Source: CAD feature listing. Evaluate the final solid. Frame: model axes, mm. Face numbers are marked on the shaded views. A direction names the side the tool comes from. Coordinates: 2 decimals unless noted, no trailing zeros. Order: outer loops, then holes, each group sorted by start corner. A loop starts at its lowest first (then second) coordinate and runs counter-clockwise, first axis right, second up.
Item 1: Section B-B on y = 0. State how many separate pieces and enclosed holes the cut face has, then the cut area to 3 significant figures.
Item 2: Section A-A on z = 22. Return the cut outline in (x, y).
Item 3: Reachability of the marked faces 1, 2 and 3 from +Z, -Z, +X, -X, +Y, -Y: full face, straight path, thin tool, end or side. Return the list, or none.
Item 4: Ray query, line 1 (Z direction, x = 1.5, y = -0.75); line 2 (X direction, y = 0, z = 2.5); line 3 (Y direction, x = -1.5, z = 19.5). Return the intervals inside material, ascending.
Item 5: Contact query for flat-ended pins moving along their axis: P1, Ø4, axis at y = -1, z = 29, coming from the +X side; P2, Ø0.6, axis at y = 1.5, z = 40, coming from the -X side; P3, Ø2.5, axis at x = 0, y = 0, coming from the -Z side; P4, Ø0.6, axis at x = 1, y = -2, coming from the -Z side. Output: stop coordinate, or through.
from build123d import *

# Parameters (mm, degrees)
SKETCH_R        = 2.5
SKETCH_R_2      = 1.6
PAD_DEPTH       = 45
PAD001_DEPTH    = 1.5
PAD002_DEPTH    = 5
SKETCH003_W     = 2
SKETCH003_H     = 7
POCKET_DEPTH    = 7.001
SKETCH004_R     = 1.1
POCKET001_DEPTH = 7.001
SKETCH006_W     = 2.5
SKETCH006_H     = 6.5
POCKET002_DEPTH = 8.001
SKETCH005_W     = 2.5
SKETCH005_H     = 6
POCKET003_DEPTH = 8.001
POCKET004_DEPTH = 7.001


with BuildPart() as part:
    # Sketch → Pad (new body)
    with BuildSketch(Plane.XY):
        Circle(SKETCH_R)
        Circle(SKETCH_R_2, mode=Mode.SUBTRACT)
    extrude(amount=PAD_DEPTH)

    # Sketch001 (on Face3 of Pad) → Pad001 (join)
    with BuildSketch(Plane(origin=(0, 0, 7), x_dir=(1, 0, 0), z_dir=(0, 0, -1))):
        with BuildLine():
            Line((-2, 4), (2, 4))
            ThreePointArc((4, 2), (3.414214, 3.414214), (2, 4))
            Line((4, 2), (4, -2))
            ThreePointArc((2, -4), (3.414214, -3.414214), (4, -2))
            Line((2, -4), (-2, -4))
            ThreePointArc((-4, -2), (-3.414214, -3.414214), (-2, -4))
            Line((-4, -2), (-4, 2))
            ThreePointArc((-2, 4), (-3.414214, 3.414214), (-4, 2))
        make_face()
    extrude(amount=-PAD001_DEPTH)

    # Sketch002 (on Face16 of Pad001) → Pad002 (join)
    with BuildSketch(Plane.XY.offset(45)):
        with BuildLine():
            Line((-1, 3), (1, 3))
            ThreePointArc((3, 1), (2.414214, 2.414214), (1, 3))
            Line((3, 1), (3, -1))
            ThreePointArc((1, -3), (2.414214, -2.414214), (3, -1))
            Line((1, -3), (-1, -3))
            ThreePointArc((-3, -1), (-2.414214, -2.414214), (-1, -3))
            Line((-3, -1), (-3, 1))
            ThreePointArc((-1, 3), (-2.414214, 2.414214), (-3, 1))
        make_face()
    extrude(amount=PAD002_DEPTH)

    # Sketch003 (on Face10 of Pad002) → Pocket (cut, through all)
    with BuildSketch(Plane.YZ.offset(3)):
        with Locations((0, 46.5)):
            Rectangle(SKETCH003_W, SKETCH003_H)
    extrude(amount=-POCKET_DEPTH, mode=Mode.SUBTRACT)

    # Sketch004 (on Face3 of Pocket) → Pocket001 (cut, through all)
    with BuildSketch(Plane.XZ.offset(3)):
        with Locations((0, 47.5)):
            Circle(SKETCH004_R)
    extrude(amount=-POCKET001_DEPTH, mode=Mode.SUBTRACT)

    # Sketch006 (on Face28 of Pocket001) → Pocket002 (cut, through all)
    with BuildSketch(Plane.XZ.offset(4)):
        with Locations((0, 13.75)):
            Rectangle(SKETCH006_W, SKETCH006_H)
        with Locations((0, 22.25)):
            Rectangle(SKETCH006_W, SKETCH006_H)
        with Locations((0, 30.75)):
            Rectangle(SKETCH006_W, SKETCH006_H)
        with Locations((0, 39.25)):
            Rectangle(SKETCH006_W, SKETCH006_H)
    extrude(amount=-POCKET002_DEPTH, mode=Mode.SUBTRACT)

    # Sketch005 (on Face31 of Pocket001) → Pocket003 (cut, through all)
    with BuildSketch(Plane.YZ.offset(4)):
        with Locations((0, 13.5)):
            Rectangle(SKETCH005_W, SKETCH005_H)
        with Locations((0, 21.5)):
            Rectangle(SKETCH005_W, SKETCH005_H)
        with Locations((0, 29.5)):
            Rectangle(SKETCH005_W, SKETCH005_H)
        with Locations((0, 37.5)):
            Rectangle(SKETCH005_W, SKETCH005_H)
    extrude(amount=-POCKET003_DEPTH, mode=Mode.SUBTRACT)

    # Sketch007 (on Face5 of Pocket003) → Pocket004 (cut, through all)
    with BuildSketch(Plane.XZ.offset(3)):
        with BuildLine():
            ThreePointArc((3, 47.251006), (2.034513, 49.208821), (0, 50))
            Line((0, 50), (3, 50))
            Line((3, 47.251006), (3, 50))
        make_face()
    extrude(amount=-POCKET004_DEPTH, mode=Mode.SUBTRACT)


solid = part.part
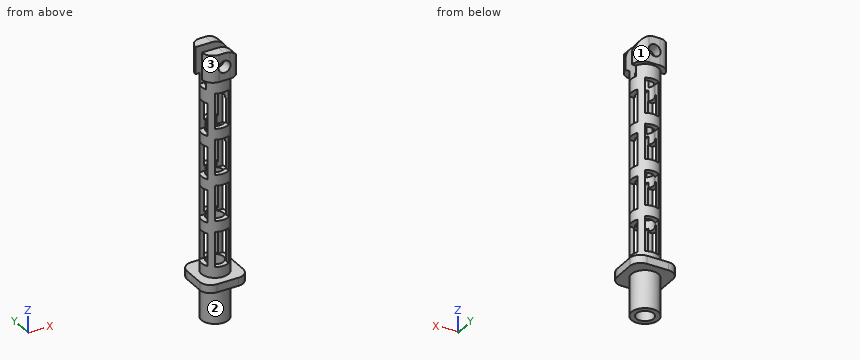
Answer list:
1. separate pieces: 9
1. enclosed holes: 0
1. area: 43.5 mm2
2. outline: (-2.17, -1.25) arc R2.5 ccw to (-1.25, -2.17) - (-1.25, -1.25) - close; (-2.17, 1.25) - (-1.25, 1.25) - (-1.25, 2.17) arc R2.5 ccw to start; (1.25, -2.17) arc R2.5 ccw to (2.17, -1.25) - (1.25, -1.25) - close; (1.25, 1.25) - (2.17, 1.25) arc R2.5 ccw to (1.25, 2.17) - close
3. face 1: +Z, +X, +Y
3. face 2: -Z
3. face 3: +Z, -X, -Y
4. line 1: z = 0 to 10.5, 16.5 to 18.5, 24.5 to 26.5, 32.5 to 34.5, 40.5 to 43
4. line 2: x = -2.5 to -1.6, 1.6 to 2.5
4. line 3: y = -2 to -1.25, 1.25 to 2
5. P1: stops at x = 2.17
5. P2: stops at x = -2.17
5. P3: stops at z = 7
5. P4: stops at z = 0
